Source: CAD feature listing. Evaluate the final solid. Frame: model axes, mm. Face numbers are marked on the shaded views. A direction names the side the tool comes from. Round coordinates to 2 decimals unless told otherwise and drop trailing zeros. Order: outer loops, then holes, each group sorted by start corner. A loop starts at its lowest first (then second) coordinate and runs counter-clockwise, first axis right, second up. Notation, with made-up numbers: M 83.5,-9 L 95.5,-9 A23 cw 95.5,16 Z; hole C 25,10.5 d5. An arc over 180 degrees is marked long. Answer as CSV lines item,"result". Start each with the question number.
Item 1: Section query C-C on y = 14. Return the cut outline in (x, z).
Item 2: Pull-direction query (X, two-part tool) for the marked faces 3, 4 and 5; classes: +X half, -X half, draft (parallel to the pull), parting line (faces both ways), or undercut.
Item 3: Set-up query: the marked faces 1 and 2. Return all of +Z, -Z, +X, -X, +Y, -Y with unobstructed straight access to the full face (end or side cutting, diameter ignored); none if empty.
Item 4: Line query: line 1 (Y direction, x = -2.5, z = -2); line 2 (Z direction, x = -13, y = 22); line 3 (X direction, y = 15.5, z = 16.5). Output: solid intervals per line, ascending. Write a range as [from, to].
Item 5: First-contact query: P1, Ø4, axis at x = 9, y = 18, coming from the -Z side (3 decimals); P2, Ø5, axis at y = 16, z = 4, coming from the -X side; P3, Ø2, axis at y = 21.5, z = -5, coming from the +X side. Flat tips, straight axial feed; report the tip coordinate or a pass-through.
Item 6: Section query A-A on x = 0. Return the cut outline in (y, z).
Item 7: Section query B-B on y = 19. Return the cut outline in (x, z), plus the area to 3 significant figures.
Autodesk Fusion 360 part; units mm, degrees
sketch "Skizze1" plane through (0, 0, 0) normal (0, 0, 1) x (1, 0, 0)
  circle A0 centre (0, 0) radius 20
  line L0 (0, 50) -> (0, -36.4171) construction
  line L1 (-20, 23) -> (20, 23)
  line L2 (20, 23) -> (20, 16.6992)
  line L3 (20, 16.6992) -> (16.0259, 11.9654)
  line L4 (-20, 23) -> (-20, 16.6992)
  line L5 (-20, 16.6992) -> (-16.0259, 11.9654)
  line L6 (-16.0259, 11.9654) -> (16.0259, 11.9654) construction
  line L7 (-18, 21) -> (18, 21)
  line L8 (18, 21) -> (18, 17.4274)
  line L9 (18, 17.4274) -> (14.7285, 13.5304)
  line L10 (-18, 21) -> (-18, 17.4274)
  line L11 (-18, 17.4274) -> (-14.7285, 13.5304)
  line L12 (0, 23) -> (0, 21)
  point P0 (0, 20)
  dimension "d1" = 40
  dimension "d2" = 40
  dimension "d3" = 3
  dimension "d4" = 2
  dimension "d5" = 2
  dimension "d6" = 2
  dimension "d7" = 2
  dimension "d8" = 2
revolve "Drehen1" add sketch "Skizze1" angle 360 about axis through (0, 50, 0) along (0, -1, 0) contours A0 L1 L4 L5 L7 L10 L11 L12
sketch "Skizze2" plane through (0, 21, 0) normal (0, -1, 0) x (1, 0, 0)
  circle A0 centre (0, 0) radius 18
  circle A1 centre (0, 0) radius 20.5
  line L0 (0, 0) -> (7.1898, 19.1978)
  line L1 (0, 0) -> (13.3222, 15.581)
  line L2 (0, 0) -> (17.8478, 10.0849)
  line L3 (0, 0) -> (20.2207, 3.3724)
  line L4 (0, 0) -> (20.1547, -3.7469)
  line L5 (0, 0) -> (0.1901, 20.4991)
  line L6 (0, 0) -> (-6.8324, 19.3279)
  line L7 (0, 0) -> (-13.0309, 15.8255)
  line L8 (0, 0) -> (-17.6577, 10.4142)
  line L9 (0, 0) -> (-20.1547, 3.7469)
  line L10 (0, 0) -> (-20.2207, -3.3724)
  line L11 (0, 0) -> (-17.8478, -10.0849)
  line L12 (0, 0) -> (-13.3222, -15.581)
  line L13 (0, 0) -> (17.6577, -10.4142)
  line L14 (0, 0) -> (13.0309, -15.8255)
  line L15 (0, 0) -> (6.8324, -19.3279)
  line L16 (0, 0) -> (-7.1898, -19.1978)
  line L17 (0, 0) -> (-0.1901, -20.4991)
  dimension "d10" = 41
  dimension "d12" = 20
  dimension "d13" = 20
  dimension "d14" = 20
  dimension "d15" = 20
  dimension "d16" = 20
  dimension "d17" = 20
  dimension "d18" = 20
  dimension "d19" = 20
  dimension "d20" = 20
  dimension "d21" = 20
  dimension "d22" = 20
  dimension "d23" = 20
  dimension "d24" = 20
  dimension "d25" = 20
  dimension "d26" = 20
  dimension "d27" = 20
  dimension "d28" = 20
extrude "Extrusion1" cut sketch "Skizze2" along normal blind 20 contours A0 L2 L3 | A0 A1 L2 L3 | A0 A1 L4 L13 | A0 L4 L13 | A0 L1 L2 | A0 A1 L1 L2 | A0 L0 L5 | A0 L5 L6 | A0 L7 L8 | A0 L8 L9 | A0 L10 L11 | A0 L11 L12 | A0 L13 L14 | A0 L16 L17 | A0 L15 L17 | A0 A1 L13 L14 | A0 A1 L0 L5 | A0 A1 L5 L6 | A0 A1 L7 L8 | A0 A1 L8 L9 | A0 A1 L10 L11 | A0 A1 L11 L12 | A0 A1 L15 L17 | A0 A1 L16 L17
fillet "Abrundung1" radius 2 6 edges at (-10.1602, 16.6992, -17.227) (9.8389, 16.6992, -17.4125) (19.9991, 16.6992, -0.1855) (-19.9991, 16.6992, 0.1855) (-9.8389, 16.6992, 17.4125) (10.1602, 16.6992, 17.227)
chamfer "Fase1" distance 0.5 angle 45 6 edges at (17.227, 21, -10.1602) (-0.1855, 21, -19.9991) (17.4125, 21, 9.8389) (0.1855, 21, 19.9991) (-17.227, 21, 10.1602) (-17.4125, 21, -9.8389)
fillet "Abrundung2" radius 1 1 edges at (-18.6465, 23, 7.2323)
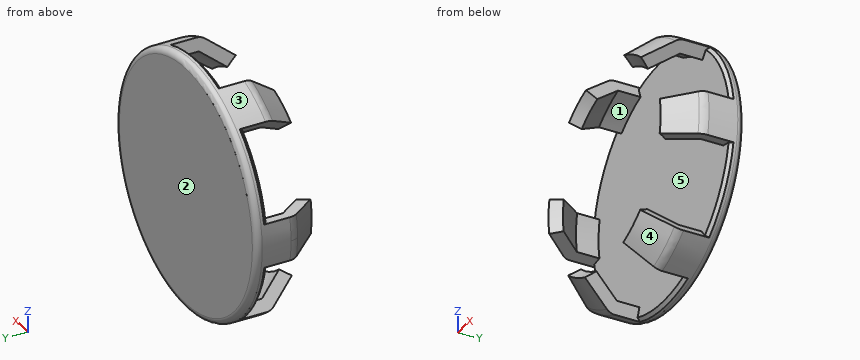
Results:
1,outline,"M -17.49,-2.92 L -14.92,-2.49 A15.12 cw -14.87,2.76 L -17.44,3.24 A17.73 ccw Z; M -11.52,-13.48 A17.73 ccw -6.22,-16.61 L -5.3,-14.16 A15.12 cw -9.83,-11.49 Z; M -11.27,13.69 L -9.61,11.67 A15.12 cw -5.04,14.26 L -5.91,16.72 A17.73 ccw Z; M 5.04,-14.26 L 5.91,-16.72 A17.73 ccw 11.27,-13.69 L 9.61,-11.67 A15.12 cw Z; M 5.3,14.16 A15.12 cw 9.83,11.49 L 11.52,13.48 A17.73 ccw 6.22,16.61 Z; M 14.87,-2.76 L 17.44,-3.24 A17.73 ccw 17.49,2.92 L 14.92,2.49 A15.12 cw Z"
2,face 3,"parting line"
2,face 4,"+X half"
2,face 5,"undercut"
3,face 1,"none"
3,face 2,"+Z, -Z, +X, -X, +Y"
4,line 1,"[21, 23]"
4,line 2,"[-15.2, 15.2]"
4,line 3,"[-9.41, -5.83], [6.18, 9.41]"
5,P1,"z = -18.735"
5,P2,"x = -19.91"
5,P3,"x = 19.6"
6,outline,"M 21,-19.5 L 21.5,-20 L 22,-20 A1 ccw 23,-19 L 23,19 A1 ccw 22,20 L 21.5,20 L 21,19.5 Z"
7,outline,"M -19.73,-3.29 L -17.75,-2.96 A18 cw -17.7,3.29 L -19.66,3.66 A20 ccw Z; M -13,-15.2 A20 ccw -7.01,-18.73 L -6.31,-16.86 A18 cw -11.7,-13.68 Z; M -12.71,15.44 L -11.44,13.9 A18 cw -6,16.97 L -6.67,18.86 A20 ccw Z; M 6,-16.97 L 6.67,-18.86 A20 ccw 12.71,-15.44 L 11.44,-13.9 A18 cw Z; M 6.31,16.86 A18 cw 11.7,13.68 L 13,15.2 A20 ccw 7.01,18.73 Z; M 17.7,-3.29 L 19.66,-3.66 A20 ccw 19.73,3.29 L 17.75,2.96 A18 cw Z"
7,area,"79.6 mm^2"
